```python
from build123d import *

# Parameters (mm, degrees)
F1_DEPTH = 3
F2_W     = 5
F2_H     = 6
F3_DEPTH = 4.775
F4_D     = 2.2
F5_R     = 2
F6_R     = 0.5


# Not quite as in the source:
# - a feature names something its author has since deleted; it is built from what else it names


with BuildPart() as f1:
    # F0 (on Front) → F1 (new body)
    with BuildSketch(Plane.XZ):
        Polygon((0.0109257422, 3), (0, 0), (14, 0), (14, 7.4), (11, 7.4), (11, 13.9), (6.25, 13.9), (6.25, 4.4), (11, 4.4), (11, 3), align=None)
    extrude(amount=F1_DEPTH)

    # F2 (on face) → F3 (join)
    with BuildSketch(Plane.YZ.offset(11)):
        with Locations((2.5, 10.9)):
            Rectangle(F2_W, F2_H)
    extrude(amount=-F3_DEPTH)

    # F4 (through all)
    with Locations(Plane.YZ.offset(11)):
        with Locations((2.5, 10.9)):
            Hole(F4_D / 2)

    # F5
    f5_edges = [f1.edges().sort_by_distance(p)[0] for p in [
        (8.6125, 5, 13.9),
        (8.6125, 5, 7.9),
        (8.625, -3, 13.9),
    ]]
    fillet(f5_edges, radius=F5_R)

    # F6 (call 1 of 5: OpenCascade refuses the feature's edges together)
    f6_edges = [f1.edges().sort_by_distance(p)[0] for p in [
        (14, -1.5, 7.4),
        (11, -1.5, 7.4),
        (11, 1, 13.9),
        (11, -3, 9.65),
        (12.5, -3, 7.4),
        (11, -2.414214, 13.314214),
        (11, 4.414214, 13.314214),
        (11, 1.5, 7.9),
        (11, 5, 10.9),
        (11, 4.414214, 8.485786),
    ]]
    fillet(f6_edges, radius=F6_R)

    # F6#2 (call 2 of 5)
    f6_2_edges = [f1.edges().sort_by_distance(p)[0] for p in [
        (6.25, -1.5, 4.4),
    ]]
    fillet(f6_2_edges, radius=F6_R)

    # F6#3 (call 3 of 5)
    f6_3_edges = [f1.edges().sort_by_distance(p)[0] for p in [
        (14, -1.5, 0),
    ]]
    fillet(f6_3_edges, radius=F6_R)

    # F6#4 (call 4 of 5)
    f6_4_edges = [f1.edges().sort_by_distance(p)[0] for p in [
        (11, -1.5, 4.4),
    ]]
    fillet(f6_4_edges, radius=F6_R)

    # F6#5 (call 5 of 5)
    f6_5_edges = [f1.edges().sort_by_distance(p)[0] for p in [
        (11, -1.5, 3),
    ]]
    fillet(f6_5_edges, radius=F6_R)

    # F7: F1 across face


with BuildPart() as f1_1:
    add(f1.part)
    add(f1.part.mirror(Plane(origin=(0.0054628711, -1.5, 1.5), x_dir=(0, -1, 0), z_dir=(-0.9999933683, 0, 0.0036418899))))


solid = f1_1.part
```
For this review, take the finished solid that the model builds, in its own axes (mm). A direction names the side the tool comes from. Round coordinates to 2 decimals unless told otherwise and drop trailing zeros. Write each loop counter-clockwise with the first axis right and the second up, starting at its lowest first coordinate (ties: lowest second). Pieces come first, ordered by that corner, then holes. Notation, with made-up numbers: (40, 65.5) -> (51, 65.5) arc R21 cw to (51, 71.5) -> close; hole circle Ø3 at (31.5, -13). An arc over 180 degrees is marked (long way). One line per question, with ' | ' between items. Start each with the question number.
(1) Add section B-B, the plane y = 2.5. Write out the cut boundary in (x, z) (3 decimals), plus the area to 3 significant figures.
(2) Tool access review of faces 1 (the face through (-8.24, 4.4, 13.39)), 2 (the face through (0, -3, 2)), 3 (the face through (13, -1, 7.4)), 4 (the face through (-8.49, 1.91, 11.89)), 5 (the face through (5, -1, 3)): name each direction out of +Z, -Z, +X, -X, +Y, -Y from which nothing blocks a thin tool from reaching the whole face with its end or side.
(3) Mouldability with a two-part tool opening along X and no side actions: class faces 6 (the face through (14, -1, 4)), 7 (the face through (8, 1, 13.9)), 8 (the face through (6.225, 1, 11)), 9 (the face through (9, -1, 4.4)) as released by +X, released by -X, zero draft, split by the parting line, or undercut.
(4) Insertion check: P1, Ø2, axis at x = 11, y = 4, coming from the -Z side; P2, Ø4, axis at y = 3.5, z = 10.5, coming from the -X side; P3, Ø2.5, axis at y = 2.5, z = 10.9, coming from the +X side; P4, Ø1, axis at x = 5, y = 3.5, coming from the +Z side. Each pin has a flat end and moves straight along its axis. Give the tip position at first contact, or say it passes through.
(5) Add section C-C, the plane z = 6. Write out the cut boundary in (x, y).
(6) Add section A-A, the plane x = 9.25. Write out the cut boundary in (y, z), plus the area to 3 significant figures.
Answer list:
1) outline: (-10.939, 8.48) arc R0.5 ccw to (-10.442, 7.976) -> (-6.167, 7.945) -> (-6.153, 9.845) -> (-10.928, 9.88) -> close; (-10.912, 12.08) -> (-6.137, 12.045) -> (-6.124, 13.945) -> (-10.398, 13.976) arc R0.5 ccw to (-10.902, 13.48) -> close; (6.225, 7.9) -> (10.5, 7.9) arc R0.5 ccw to (11, 8.4) -> (11, 9.8) -> (6.225, 9.8) -> close; (6.225, 12) -> (11, 12) -> (11, 13.4) arc R0.5 ccw to (10.5, 13.9) -> (6.225, 13.9) -> close | area: 36.1 mm²
2) face 1: +Z, +X, +Y | face 2: +Z, -Z, +X, -X, -Y | face 3: +Z, +X, +Y, -Y | face 4: none | face 5: +Y, -Y
3) face 6: released by +X | face 7: zero draft | face 8: undercut | face 9: undercut
4) P1: z = 7.9 | P2: x = -10.94 | P3: x = 11 | P4: through
5) outline: (-13.96, -3) -> (-6.21, -3) -> (-6.21, 0) -> (-13.96, 0) -> close; (6.25, -3) -> (14, -3) -> (14, 0) -> (6.25, 0) -> close
6) outline: (-3, 0) -> (0, 0) -> (0, 3) -> (-3, 3) -> close; (-3, 4.4) -> (0, 4.4) -> (0, 7.9) -> (3, 7.9) arc R2 ccw to (5, 9.9) -> (5, 11.9) arc R2 ccw to (3, 13.9) -> (-1, 13.9) arc R2 ccw to (-3, 11.9) -> close; hole circle Ø2.2 at (2.5, 10.9) | area: 61.1 mm²
